```python
from build123d import *

# Parameters (mm, degrees)
RESSALTO_EXTRUS_O1_DEPTH = 7
CORTE_EXTRUS_O1_DEPTH    = 31.512292605
RESSALTO_EXTRUS_O2_DEPTH = 3
ESBO_O4_R                = 1.7
RESSALTO_EXTRUS_O3_DEPTH = 1.6
CORTE_EXTRUS_O2_REACH    = 49.476
ESBO_O5_W                = 10.45
ESBO_O5_H                = 6
ESBO_O6_W                = 10.45
ESBO_O6_H                = 24
RESSALTO_EXTRUS_O4_DEPTH = 1
CORTE_EXTRUS_O3_REACH    = 32.512
ESBO_O8_R                = 1.6
ESBO_O11_R               = 2.9
CORTE_EXTRUS_O4_DEPTH    = 5
RESSALTO_EXTRUS_O5_DEPTH = 22


with BuildPart() as part:
    # Esboço1 → Ressalto-extrusão1 (new body)
    with BuildSketch(Plane.XY):
        with BuildLine():
            Line((15.5, -21), (-15.5, -21))
            ThreePointArc((-15.5, -21), (-19.389087297, -19.389087297), (-21, -15.5))
            Line((-21, -15.5), (-21, 15.5))
            ThreePointArc((-21, 15.5), (-19.389087297, 19.389087297), (-15.5, 21))
            Line((-15.5, 21), (15.5, 21))
            ThreePointArc((15.5, 21), (19.389087297, 19.389087297), (21, 15.5))
            Line((21, 15.5), (21, -15.5))
            ThreePointArc((21, -15.5), (19.389087297, -19.389087297), (15.5, -21))
        make_face()
    extrude(amount=RESSALTO_EXTRUS_O1_DEPTH)

    # Esboço2 → Corte-extrusão1 (cut, through all)
    with BuildSketch(Plane(origin=(0, 0, 0), x_dir=(-1, 0, 0), z_dir=(0, 0, -1))):
        with BuildLine():
            Line((10, -12), (-10, -12))
            ThreePointArc((-10, -12), (-11.414213562, -11.414213562), (-12, -10))
            Line((-12, -10), (-12, 10))
            ThreePointArc((-12, 10), (-11.414213562, 11.414213562), (-10, 12))
            Line((-10, 12), (10, 12))
            ThreePointArc((10, 12), (11.414213562, 11.414213562), (12, 10))
            Line((12, 10), (12, -10))
            ThreePointArc((12, -10), (11.414213562, -11.414213562), (10, -12))
        make_face()
    extrude(amount=-CORTE_EXTRUS_O1_DEPTH, mode=Mode.SUBTRACT)

    # Esboço3 → Ressalto-extrusão2 (add)
    with BuildSketch(Plane(origin=(0, 0, 0), x_dir=(-1, 0, 0), z_dir=(0, 0, -1))):
        with BuildLine():
            Line((-5.225, 12), (-5.225, -12))
            Line((-5.225, -12), (-10, -12))
            ThreePointArc((-10, -12), (-11.414213562, -11.414213562), (-12, -10))
            Line((-12, -10), (-12, 10))
            ThreePointArc((-12, 10), (-11.414213562, 11.414213562), (-10, 12))
            Line((-10, 12), (-5.225, 12))
        make_face()
        with BuildLine():
            Line((5.225, 12), (10, 12))
            ThreePointArc((10, 12), (11.414213562, 11.414213562), (12, 10))
            Line((12, 10), (12, -10))
            ThreePointArc((12, -10), (11.414213562, -11.414213562), (10, -12))
            Line((10, -12), (5.225, -12))
            Line((5.225, -12), (5.225, 12))
        make_face()
    extrude(amount=-RESSALTO_EXTRUS_O2_DEPTH)

    # Esboço4 → Ressalto-extrusão3 (add)
    with BuildSketch(Plane.XY.offset(3)):
        with Locations((-8, 8)):
            Circle(ESBO_O4_R)
        with Locations(Location((8, 8, 0), (0, 0, 180))):
            Circle(ESBO_O4_R)
        with Locations(Location((8, -8, 0), (0, 0, 180))):
            Circle(ESBO_O4_R)
        with Locations((-8, -8)):
            Circle(ESBO_O4_R)
    extrude(amount=RESSALTO_EXTRUS_O3_DEPTH)

    # Esboço5 → Corte-extrusão2 (cut, up to next)
    with BuildSketch(Plane.XZ.offset(21), mode=Mode.PRIVATE) as corte_extrus_o2_sk1:
        with Locations((0, 4)):
            Rectangle(ESBO_O5_W, ESBO_O5_H)
    corte_extrus_o2_tool1 = extrude(corte_extrus_o2_sk1.sketch, amount=-CORTE_EXTRUS_O2_REACH, mode=Mode.PRIVATE) & part.part
    add(corte_extrus_o2_tool1.solids().sort_by_distance((0, -21, 4))[0], mode=Mode.SUBTRACT)

    # Esboço6 → Ressalto-extrusão4 (add)
    with BuildSketch(Plane(origin=(0, 0, 0), x_dir=(-1, 0, 0), z_dir=(0, 0, -1))):
        Rectangle(ESBO_O6_W, ESBO_O6_H)
    extrude(amount=-RESSALTO_EXTRUS_O4_DEPTH)

    # Esboço8 → Corte-extrusão3 (cut, up to next)
    with BuildSketch(Plane.XY.offset(7), mode=Mode.PRIVATE) as corte_extrus_o3_sk1:
        with Locations((-15.5, 15.5)):
            Circle(ESBO_O8_R)
    corte_extrus_o3_tool1 = extrude(corte_extrus_o3_sk1.sketch, amount=-CORTE_EXTRUS_O3_REACH, mode=Mode.PRIVATE) & part.part
    # Esboço8 → Corte-extrusão3 (cut, up to next)
    with BuildSketch(Plane.XY.offset(7), mode=Mode.PRIVATE) as corte_extrus_o3_sk2:
        with Locations(Location((15.5, 15.5, 0), (0, 0, 180))):
            Circle(ESBO_O8_R)
    corte_extrus_o3_tool2 = extrude(corte_extrus_o3_sk2.sketch, amount=-CORTE_EXTRUS_O3_REACH, mode=Mode.PRIVATE) & part.part
    # Esboço8 → Corte-extrusão3 (cut, up to next)
    with BuildSketch(Plane.XY.offset(7), mode=Mode.PRIVATE) as corte_extrus_o3_sk3:
        with Locations((15.5, -15.5)):
            Circle(ESBO_O8_R)
    corte_extrus_o3_tool3 = extrude(corte_extrus_o3_sk3.sketch, amount=-CORTE_EXTRUS_O3_REACH, mode=Mode.PRIVATE) & part.part
    # Esboço8 → Corte-extrusão3 (cut, up to next)
    with BuildSketch(Plane.XY.offset(7), mode=Mode.PRIVATE) as corte_extrus_o3_sk4:
        with Locations(Location((-15.5, -15.5, 0), (0, 0, 180))):
            Circle(ESBO_O8_R)
    corte_extrus_o3_tool4 = extrude(corte_extrus_o3_sk4.sketch, amount=-CORTE_EXTRUS_O3_REACH, mode=Mode.PRIVATE) & part.part
    add(corte_extrus_o3_tool1.solids().sort_by_distance((-15.5, 15.5, 7))[0], mode=Mode.SUBTRACT)
    add(corte_extrus_o3_tool2.solids().sort_by_distance((15.5, 15.5, 7))[0], mode=Mode.SUBTRACT)
    add(corte_extrus_o3_tool3.solids().sort_by_distance((15.5, -15.5, 7))[0], mode=Mode.SUBTRACT)
    add(corte_extrus_o3_tool4.solids().sort_by_distance((-15.5, -15.5, 7))[0], mode=Mode.SUBTRACT)

    # Esboço11 → Corte-extrusão4 (cut)
    with BuildSketch(Plane(origin=(0, 0, 0), x_dir=(-1, 0, 0), z_dir=(0, 0, -1))):
        with Locations((-15.5, 15.5)):
            Circle(ESBO_O11_R)
        with Locations(Location((15.5, 15.5, 0), (0, 0, 180))):
            Circle(ESBO_O11_R)
        with Locations((15.5, -15.5)):
            Circle(ESBO_O11_R)
        with Locations(Location((-15.5, -15.5, 0), (0, 0, 180))):
            Circle(ESBO_O11_R)
    extrude(amount=-CORTE_EXTRUS_O4_DEPTH, mode=Mode.SUBTRACT)

    # Esboço13 → Ressalto-extrusão5 (add)
    with BuildSketch(Plane(origin=(0, 0, 0), x_dir=(-1, 0, 0), z_dir=(0, 0, -1))):
        with BuildLine():
            Line((24, -15.5), (24, 15.5))
            ThreePointArc((24, 15.5), (21.51040764, 21.51040764), (15.5, 24))
            Line((15.5, 24), (-15.5, 24))
            ThreePointArc((-15.5, 24), (-21.51040764, 21.51040764), (-24, 15.5))
            Line((-24, 15.5), (-24, -15.5))
            ThreePointArc((-24, -15.5), (-21.51040764, -21.51040764), (-15.5, -24))
            Line((-15.5, -24), (-11.5, -24))
            Line((-11.5, -24), (-11.5, -21))
            Line((-11.5, -21), (-15.5, -21))
            ThreePointArc((-15.5, -21), (-19.389087297, -19.389087297), (-21, -15.5))
            Line((-21, -15.5), (-21, 15.5))
            ThreePointArc((-21, 15.5), (-19.389087297, 19.389087297), (-15.5, 21))
            Line((-15.5, 21), (15.5, 21))
            ThreePointArc((15.5, 21), (19.389087297, 19.389087297), (21, 15.5))
            Line((21, 15.5), (21, -15.5))
            ThreePointArc((21, -15.5), (19.389087297, -19.389087297), (15.5, -21))
            Line((15.5, -21), (11.5, -21))
            Line((11.5, -21), (11.5, -24))
            Line((11.5, -24), (15.5, -24))
            ThreePointArc((15.5, -24), (21.51040764, -21.51040764), (24, -15.5))
        make_face()
    extrude(amount=-RESSALTO_EXTRUS_O5_DEPTH)


solid = part.part
```
The listing builds one solid part. Answer for the finished solid, in the listing's coordinates (mm). A direction names the side the tool comes from. Coordinates: 2 decimals unless noted, no trailing zeros. Order: outer loops, then holes, each group sorted by start corner. A loop starts at its lowest first (then second) coordinate and runs counter-clockwise, first axis right, second up. Notation, with made-up numbers: M 56.25,-10 L 89.25,-10 A34 cw 89.25,24 Z; hole C 76,56.25 d8. An arc over 180 degrees is marked long. Answer as a JSON object with one key per item and string values. Group by question number.
1. Section B-B on y = 8 is taken. Write down the section's boundary in (x, z) (3 decimals), then the cut area to 3 significant figures.
2. Straight lines are drawn through the part: line 1 (Y direction, x = 15.5, z = 5.4); line 2 (Y direction, x = 15.5, z = 1.9); line 3 (X direction, y = 12.5, z = 15). For each, find the intervals that lie inside material, in ascending order.
3. Section D-D on y = 19.5 is taken. Write down the section's boundary in (x, z), then the cut area to 3 significant figures.
4. Section A-A on x = -4 is taken. Write down the section's boundary in (y, z), then the cut area to 3 significant figures.
5. Determine the mould class of faces 1 (the flat face through (24, 0, 11)), 2 (the flat face through (0, 24, 11)), 3 (the flat face through (5.225, -7.9, 2.6)) for opening direction X: released by +X, released by -X, zero draft, split by the parting line, or undercut.
6. Section C-C on z = 12.5 is taken. Write down the section's boundary in (x, y), then the cut area to 3 significant figures.
7. A tool of negligible diameter and unlimited length cuts with its end or side. For faces 4 (the cylindrical face through (17.801, 13.735, 2.465)), 5 (the flat face through (21, 0, 14)), 6 (the flat face through (-24, 0, 11)), 7 (the flat face through (0.2, -21, 0.3)), 8 (the flat face through (-5.225, -8.4, 2.6)), from which of +Z, -Z, +X, -X, +Y, -Y can it reach the whole face along a straight path? Write none if from no direction.
8. Flat-ended cylindrical pins translate along their axes: P1, Ø1.7, axis at x = 15, y = -14.5, coming from the -Z side; P2, Ø12, axis at x = -3, y = -9.5, coming from the +Z side; P3, Ø5, axis at x = 4.5, z = 17.5, coming from the -Y side; P4, Ø3, axis at x = -16, z = 3.5, coming from the +Y side. Find the tip coordinate at first contact, or state that the pin passes through.
Values follow:
{
 "1": {"outline": "M -24,0 L 24,0 L 24,22 L 21,22 L 21,7 L 12,7 L 12,3 L 9.7,3 L 9.7,4.6 L 6.3,4.6 L 6.3,3 L 5.225,3 L 5.225,1 L -5.225,1 L -5.225,3 L -6.3,3 L -6.3,4.6 L -9.7,4.6 L -9.7,3 L -12,3 L -12,7 L -21,7 L -21,22 L -24,22 Z", "area": "320 mm2"},
 "2": {"line 1": "-24 to -17.1, -13.9 to 13.9, 17.1 to 24", "line 2": "-24 to -18.4, -12.6 to 12.6, 18.4 to 24", "line 3": "-24 to -21, 21 to 24"},
 "3": {"outline": "M -23,0 L 23,0 L 23,22 L 19.27,22 L 19.27,7 L -19.27,7 L -19.27,22 L -23,22 Z", "area": "434 mm2"},
 "4": {"outline": "M -21,0 L 24,0 L 24,22 L 21,22 L 21,7 L 12,7 L 12,1 L -21,1 Z", "area": "162 mm2"},
 "5": {"face 1": "released by +X", "face 2": "zero draft", "face 3": "undercut"},
 "6": {"outline": "M -24,-15.5 A8.5 ccw -15.5,-24 L -11.5,-24 L -11.5,-21 L -15.5,-21 A5.5 cw -21,-15.5 L -21,15.5 A5.5 cw -15.5,21 L 15.5,21 A5.5 cw 21,15.5 L 21,-15.5 A5.5 cw 15.5,-21 L 11.5,-21 L 11.5,-24 L 15.5,-24 A8.5 ccw 24,-15.5 L 24,15.5 A8.5 ccw 15.5,24 L -15.5,24 A8.5 ccw -24,15.5 Z", "area": "435 mm2"},
 "7": {"face 4": "-Z", "face 5": "+Z", "face 6": "+Z, -Z, -X, +Y, -Y", "face 7": "+Z, -Z, -Y", "face 8": "+Z, -Y"},
 "8": {"P1": "z = 5", "P2": "z = 7", "P3": "y = 21", "P4": "y = 24"}
}
